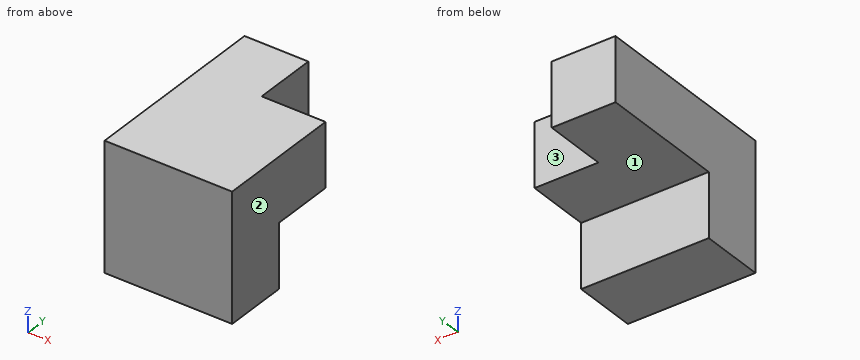
```python
from build123d import *

# Parameters (mm, degrees)
F0_W     = 12
F0_H     = 12
F1_DEPTH = 12
F2_W     = 24
F2_H     = 12
F3_DEPTH = 12
F4_W     = 24
F4_H     = 12
F5_DEPTH = 12
F6_W     = 12
F6_H     = 12
F7_DEPTH = 12


with BuildPart() as f1:
    # F0 (on Top) → F1 (new body)
    with BuildSketch(Plane.XY):
        with Locations((-35.581973, -40.582312)):
            Rectangle(F0_W, F0_H)
        with Locations((-23.581973, -40.582312)):
            Rectangle(F0_W, F0_H)
    extrude(amount=F1_DEPTH)

    # F2 (on face) → F3 (join)
    with BuildSketch(Plane.XY.offset(12)):
        with Locations((-29.581973, -40.582312)):
            Rectangle(F2_W, F2_H)
    extrude(amount=F3_DEPTH)

    # F4 (on face) → F5 (join)
    with BuildSketch(Plane(origin=(0, -34.582312, 0), x_dir=(-1, 0, 0), z_dir=(0, 1, 0))):
        with Locations((29.581973, 18)):
            Rectangle(F4_W, F4_H)
    extrude(amount=F5_DEPTH)

    # F6 (on face) → F7 (join)
    with BuildSketch(Plane(origin=(0, -22.582312, 0), x_dir=(-1, 0, 0), z_dir=(0, 1, 0))):
        with Locations((35.581973, 18)):
            Rectangle(F6_W, F6_H)
    extrude(amount=F7_DEPTH)


solid = f1.part
```
Here's how the part is built. I have some questions about the finished solid (model axes, mm). Face numbers are marked on the shaded views. A direction names the side the tool comes from. Coordinates: 2 decimals unless noted, no trailing zeros. Loops run counter-clockwise (first coordinate to the right, second up) from the corner with the lowest first, then second, coordinate; pieces in that order, holes last. Notation, with made-up numbers: (9.5, -26) - (43.5, -26) arc R32 ccw to (43.5, 10) - close; hole circle Ø8 at (-16.75, 24). An arc over 180 degrees is marked (long way). Answer as CSV lines item,"result".
Q1. For the marked faces 1, 2 and 3, which set-ups out of +Z, -Z, +X, -X, +Y, -Y let a thin tool reach every point of the face, with its end or its side?
Response:
face 1,"-Z, +X, -X, +Y"
face 2,"+Z, -Z, +X, +Y, -Y"
face 3,"+Z, -Z, +X, +Y"
Q2. If we section it at B-B, the plane x = -39.5: Write out the boundary of the cut face in (y, z).
Response:
outline,"(-46.58, 0) - (-34.58, 0) - (-34.58, 12) - (-10.58, 12) - (-10.58, 24) - (-46.58, 24) - close"
Q3. If I drill on L1, parallel to Y at x = -21.25, z = 6.75; L2, parallel to Z at x = -31, y = -24; L3, parallel to Y at x = -25.25, z = 22.5, over which ranges is the centre line in solid material (lowest first)? Write a range as [from, to].
Response:
L1,"[-46.58, -34.58]"
L2,"[12, 24]"
L3,"[-46.58, -22.58]"
Q4. For pin 1 (6 mm diameter, centred on x = -35, z = 8.5, fed in from +Y); pin 2 (13 mm diameter, centred on y = -14, z = 15.5, fed in from +X); pin 3 (6 mm diameter, centred on x = -24, z = 16.5, fed in from +Y), each with a flat end and sliding along its axis, tell me the tip position at first contact or that it passes through.
Response:
pin 1,"y = -34.58"
pin 2,"x = -29.58"
pin 3,"y = -22.58"
Q5. If we section it at D-D, the plane y = -24.5: Write out the boundary of the cut face in (x, z).
Response:
outline,"(-41.58, 12) - (-17.58, 12) - (-17.58, 24) - (-41.58, 24) - close"
Q6. If we section it at C-C, the plane y = -17: Write out the boundary of the cut face in (x, z).
Response:
outline,"(-41.58, 12) - (-29.58, 12) - (-29.58, 24) - (-41.58, 24) - close"
Q7. If we section it at A-A, the plane z = 15.25: Write out the boundary of the cut face in (x, y).
Response:
outline,"(-41.58, -46.58) - (-17.58, -46.58) - (-17.58, -22.58) - (-29.58, -22.58) - (-29.58, -10.58) - (-41.58, -10.58) - close"
